Could you check a few things on this drawing? It's one solid part, dimensions in mm from its lowest x, y, z. A direction names the side the tool comes from. Coordinates: 2 decimals unless noted, no trailing zeros. Write each loop counter-clockwise with the first axis right and the second up, starting at its lowest first coordinate (ties: lowest second). Pieces come first, ordered by that corner, then holes.
Item 1: I want a section at A-A (z = 52). Please give me the cut outline in (x, y).
Item 2: For the marked faces 1, 2 and 3, which set-ups out of +Z, -Z, +X, -X, +Y, -Y let a thin tool reach every point of the face, with its end or its side?
Item 3: I want a section at D-D (z = 84). Please give me the cut outline in (x, y), and give its area (3 significant figures).
Item 4: Please list where these lines run through material, in increasing order: line 1 (X direction, y = 28, z = 48); line 2 (Z direction, x = 179.5, y = 12); line 3 (X direction, y = 12, z = 86).
Item 5: I want a section at B-B (y = 18). Please give me the cut outline in (x, z).
Item 6: I want a section at C-C (x = 112.5). Please give me the cut outline in (y, z), and give its area (4 significant figures).
Item 7: I'm going to push flat-ended pins straight in: P1, Ø10, axis at x = 158, y = 18, coming from the +Z side; P2, Ø4, axis at x = 106, y = 11.5, coming from the -Z side; P3, Ø6, axis at y = 18, z = 87.5, coming from the +X side. Where does each tip first touch, or does it pass through?
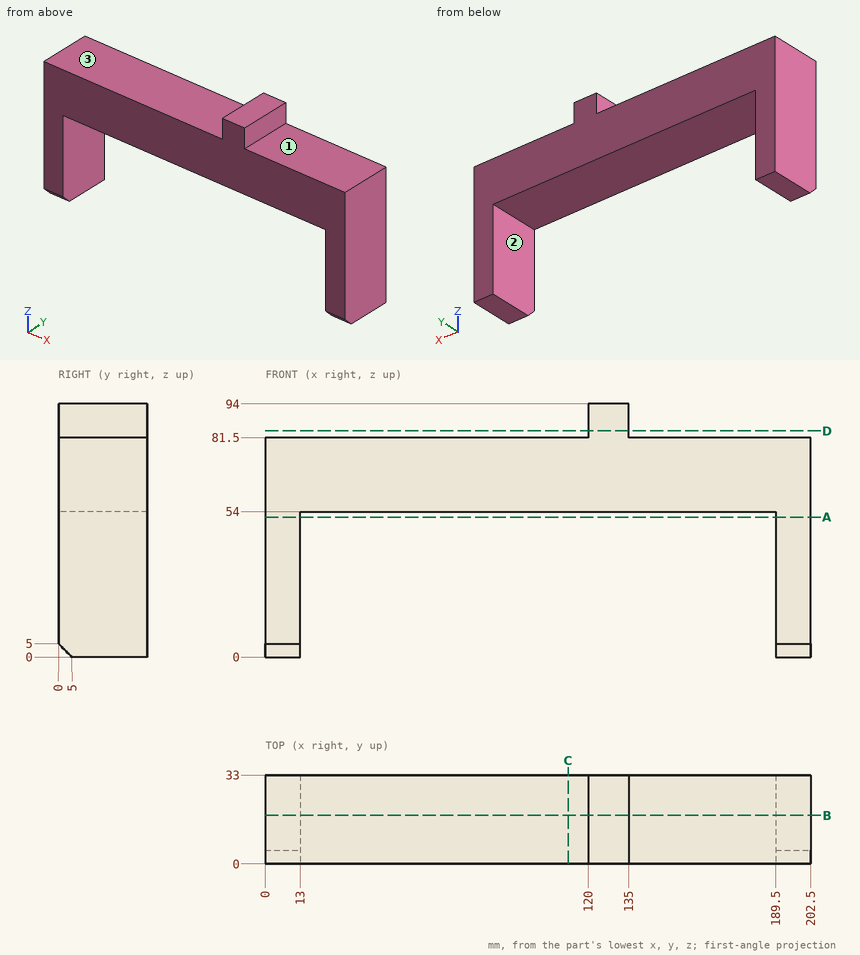
Answer:
1. outline: (0, 0) - (13, 0) - (13, 33) - (0, 33) - close; (189.5, 0) - (202.5, 0) - (202.5, 33) - (189.5, 33) - close
2. face 1: +Z, +X, +Y, -Y
2. face 2: -Z, +Y, -Y
2. face 3: +Z, -X, +Y, -Y
3. outline: (120, 0) - (135, 0) - (135, 33) - (120, 33) - close
3. area: 495 mm2
4. line 1: x = 0 to 13, 189.5 to 202.5
4. line 2: z = 54 to 81.5
4. line 3: x = 120 to 135
5. outline: (0, 0) - (13, 0) - (13, 54) - (189.5, 54) - (189.5, 0) - (202.5, 0) - (202.5, 81.5) - (135, 81.5) - (135, 94) - (120, 94) - (120, 81.5) - (0, 81.5) - close
6. outline: (0, 54) - (33, 54) - (33, 81.5) - (0, 81.5) - close
6. area: 907.5 mm2
7. P1: stops at z = 81.5
7. P2: stops at z = 54
7. P3: stops at x = 135
